For this review, take the finished solid that the model builds, in its own axes (mm). Face numbers are marked on the shaded views. Give positions to 0.01 mm unless a question says otherwise; leave off trailing zeros. Order: outer loops, then holes, each group sorted by start corner. A loop starts at its lowest first (then second) coordinate and runs counter-clockwise, first axis right, second up.
Autodesk Inventor part; units mm, degrees
ref_plane "YZ Plane" through (0, 0, 0) normal (1, 0, 0) x (0, 1, 0)
ref_plane "XZ Plane" through (0, 0, 0) normal (0, 1, 0) x (-1, 0, 0)
ref_plane "XY Plane" through (0, 0, 0) normal (0, 0, 1) x (1, 0, 0)
sketch "Sketch1" plane through (0, 0, 0) normal (0, 0, 1) x (1, 0, 0)
  line L0 (0, 0) -> (-8, 0)
  line L1 (-8, 0) -> (-8, 10)
  line L2 (-8, 10) -> (0, 10)
  line L3 (0, 10) -> (0, 0)
  dimension "d2" = 10
  dimension "d3" = 8
extrude "Extrusion1" add sketch "Sketch1" along normal blind 0.5
sketch "Sketch2" plane through (0, 0, 0) normal (1, 0, 0) x (0, 0, -1)
  line L0 (-0.5, 10) -> (-0.5, 11)
  arc A0 (0, 10) -> (-0.5, 11) centre (0.4916, 10.8708) ccw
  line L1 (0, 10) -> (-0.5, 10)
  line L2 (0, 10) -> (-0.5, 10)
  point P0 (0, 0)
  dimension "d4" = 1
  dimension "d5" = 1
extrude "Extrusion2" add sketch "Sketch2" against normal blind 8
sketch "Sketch3" plane through (0, 0, 0.5) normal (1, 0, 0) x (0, 0, -1)
  arc A0 (0.5, 10) -> (0, 11) centre (0.9916, 10.8708) ccw
  circle A1 centre (0.9916, 10.8708) radius 0.75
  point P0 (0.5, 0)
  dimension "d8" = 1.5
extrude "Extrusion3" cut sketch "Sketch3" against normal blind 8
chamfer "Chamfer1" distance 2 angle 45 2 edges at (-8, 0, 0.25) (0, 0, 0.25)
properties part number "Bottom_Trava"
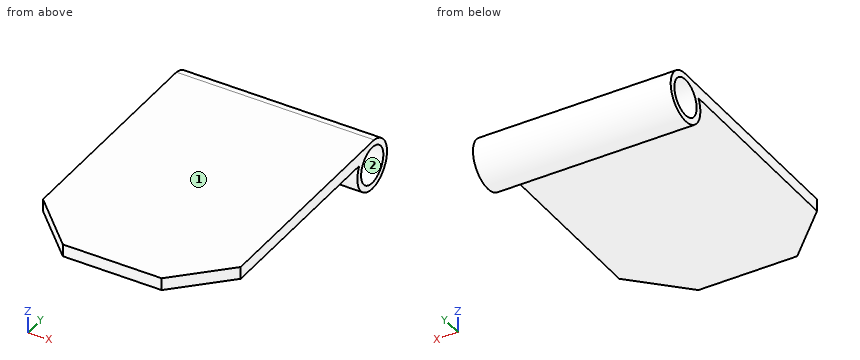
1) We need section A-A on z = -0.6. Give the boundary of the cut face in (x, y), then the cut area to 3 significant figures.
Answer sheet:
outline: (-8, 9.88) - (0, 9.88) - (0, 10.13) - (-8, 10.13) - close; (-8, 11.61) - (0, 11.61) - (0, 11.86) - (-8, 11.86) - close
area: 4.03 mm2
2) To check wall thickness, follow line 1 (Z direction, x = -3.75, y = 9); line 2 (Y direction, x = -5.5, z = -0.2); line 3 (Y direction, x = -6, z = -0.05). State the ranges of each line that lie inside material, in increasing order.
Answer sheet:
line 1: z = 0 to 0.5
line 2: y = 9.91 to 10.18, 11.56 to 11.83
line 3: y = 9.97 to 10.26, 11.48 to 11.77
3) We need section B-B on x = -2.25. Give the boundary of the cut face in (y, z).
Answer sheet:
outline: (0, 0) - (10, 0) arc R1 ccw (long way) to (11, 0.5) - (0, 0.5) - close; hole circle Ø1.5 at (10.87, -0.49)
4) We need section C-C on y = 4.75. Give the boundary of the cut face in (x, z).
Answer sheet:
outline: (-8, 0) - (0, 0) - (0, 0.5) - (-8, 0.5) - close
5) Draft analysis for pull direction Z (two halves, no side actions). For the marked faces 1 and 2, state which applies: +Z half, -Z half, draft (parallel to the pull), parting line (faces both ways), or undercut.
Answer sheet:
face 1: +Z half
face 2: undercut
6) We need section D-D on x = -1. Give the boundary of the cut face in (y, z), then the cut area to 3 significant figures.
Answer sheet:
outline: (1, 0) - (10, 0) arc R1 ccw (long way) to (11, 0.5) - (1, 0.5) - close; hole circle Ø1.5 at (10.87, -0.49)
area: 5.99 mm2
7) Clearance check with a flat-ended pin moving along its axis: pin 1 (3 mm diameter, centred on x = -1, y = 2, fed in from -Z). State where the tip first meets the part, or that it passes through.
Answer sheet:
pin 1: stops at z = 0
